from build123d import *

# Parameters (mm, degrees)
BOX319_W                    = 6
BOX319_H                    = 8
BOX319_DEPTH                = 2
BOX319_PLACEMENT_ANGLE      = 45
BOX321_W                    = 6
BOX321_H                    = 8
BOX321_DEPTH                = 2
BOX312_W                    = 6
BOX312_H                    = 8
BOX312_DEPTH                = 2
BOX324_W                    = 6
BOX324_H                    = 8
BOX324_DEPTH                = 2
BOX324_PLACEMENT_ANGLE      = 135
BOX322_W                    = 6
BOX322_H                    = 8
BOX322_DEPTH                = 2
BOX326_W                    = 6
BOX326_H                    = 8
BOX326_DEPTH                = 2
BOX326_PLACEMENT_ANGLE      = 225
BOX315_W                    = 6
BOX315_H                    = 8
BOX315_DEPTH                = 2
BOX325_W                    = 6
BOX325_H                    = 8
BOX325_DEPTH                = 2
BOX325_PLACEMENT_ANGLE      = 45
COMPOUND700_PLACEMENT_ANGLE = 22.5
CYLINDER700_R               = 1.5
CYLINDER700_DEPTH           = 12
CYLINDER700_PLACEMENT_ANGLE = 45
CYLINDER708_R               = 1.5
CYLINDER708_DEPTH           = 12
CYLINDER706_R               = 1.5
CYLINDER706_DEPTH           = 12
CYLINDER706_PLACEMENT_ANGLE = 135
CYLINDER705_R               = 1.5
CYLINDER705_DEPTH           = 12
CYLINDER707_R               = 1.5
CYLINDER707_DEPTH           = 12
CYLINDER707_PLACEMENT_ANGLE = 225
CYLINDER704_R               = 1.5
CYLINDER704_DEPTH           = 12
CYLINDER699_R               = 1.5
CYLINDER699_DEPTH           = 12
CYLINDER699_PLACEMENT_ANGLE = 45
CYLINDER702_R               = 1.5
CYLINDER702_DEPTH           = 12
COMPOUND701_PLACEMENT_ANGLE = 22.5
CYLINDER697_R               = 3.5
CYLINDER697_DEPTH           = 20
TUBE076_R                   = 46
TUBE076_R_2                 = 36
TUBE076_DEPTH               = 1


with BuildPart() as krychle319:
    # Box319 → Box319 (new body)
    with BuildSketch(Plane.XY):
        with Locations((3, 4)):
            Rectangle(BOX319_W, BOX319_H)
    extrude(amount=BOX319_DEPTH)


with BuildPart() as krychle319_1:
    # Box319 placement: moved
    add(krychle319.part.moved(Location((30.405592, -34.648232, 33))).rotate(Axis((30.405592, -34.648232, 33), (0, 0, 1)), BOX319_PLACEMENT_ANGLE))


with BuildPart() as krychle321:
    # Box321 → Box321 (new body)
    with BuildSketch(Plane(origin=(46, -3, 33), x_dir=(0, 1, 0), z_dir=(0, 0, 1))):
        with Locations((3, 4)):
            Rectangle(BOX321_W, BOX321_H)
    extrude(amount=BOX321_DEPTH)


with BuildPart() as krychle312:
    # Box312 → Box312 (new body)
    with BuildSketch(Plane(origin=(-3, -46, 33), x_dir=(1, 0, 0), z_dir=(0, 0, 1))):
        with Locations((3, 4)):
            Rectangle(BOX312_W, BOX312_H)
    extrude(amount=BOX312_DEPTH)


with BuildPart() as krychle324:
    # Box324 → Box324 (new body)
    with BuildSketch(Plane.XY):
        with Locations((3, 4)):
            Rectangle(BOX324_W, BOX324_H)
    extrude(amount=BOX324_DEPTH)


with BuildPart() as krychle324_1:
    # Box324 placement: moved
    add(krychle324.part.moved(Location((34.648232, 30.405592, 33))).rotate(Axis((34.648232, 30.405592, 33), (0, 0, 1)), BOX324_PLACEMENT_ANGLE))


with BuildPart() as krychle322:
    # Box322 → Box322 (new body)
    with BuildSketch(Plane(origin=(3, 46, 33), x_dir=(-1, 0, 0), z_dir=(0, 0, 1))):
        with Locations((3, 4)):
            Rectangle(BOX322_W, BOX322_H)
    extrude(amount=BOX322_DEPTH)


with BuildPart() as krychle326:
    # Box326 → Box326 (new body)
    with BuildSketch(Plane.XY):
        with Locations((3, 4)):
            Rectangle(BOX326_W, BOX326_H)
    extrude(amount=BOX326_DEPTH)


with BuildPart() as krychle326_1:
    # Box326 placement: moved
    add(krychle326.part.moved(Location((-30.405592, 34.648232, 33))).rotate(Axis((-30.405592, 34.648232, 33), (0, 0, 1)), BOX326_PLACEMENT_ANGLE))


with BuildPart() as krychle315:
    # Box315 → Box315 (new body)
    with BuildSketch(Plane(origin=(-46, 3, 33), x_dir=(0, -1, 0), z_dir=(0, 0, 1))):
        with Locations((3, 4)):
            Rectangle(BOX315_W, BOX315_H)
    extrude(amount=BOX315_DEPTH)


with BuildPart() as compound700:
    # Box325 → Box325 (new body)
    with BuildSketch(Plane.XY):
        with Locations((3, 4)):
            Rectangle(BOX325_W, BOX325_H)
    extrude(amount=BOX325_DEPTH)


with BuildPart() as compound700_1:
    # Box325 placement: moved
    add(compound700.part.moved(Location((-34.648232, -30.405592, 33))).rotate(Axis((-34.648232, -30.405592, 33), (0, 0, -1)), BOX325_PLACEMENT_ANGLE))

    # Compound700: union Krychle319, Krychle321, Krychle312, Krychle324, Krychle322, Krychle326, Krychle315
    add(krychle319_1.part)
    add(krychle321.part)
    add(krychle312.part)
    add(krychle324_1.part)
    add(krychle322.part)
    add(krychle326_1.part)
    add(krychle315.part)


with BuildPart() as compound700_2:
    # Compound700 placement: moved
    add(compound700_1.part.rotate(Axis((0, 0, 0), (0, 0, 1)), COMPOUND700_PLACEMENT_ANGLE))


with BuildPart() as obj1:
    # Cylinder700 → Cylinder700 (new body)
    with BuildSketch(Plane.XY):
        Circle(CYLINDER700_R)
    extrude(amount=CYLINDER700_DEPTH)


with BuildPart() as obj1_1:
    # Cylinder700 placement: moved
    add(obj1.part.moved(Location((29.698485, -29.698485, 33.5))).rotate(Axis((29.698485, -29.698485, 33.5), (0, 0, 1)), CYLINDER700_PLACEMENT_ANGLE))


with BuildPart() as obj2:
    # Cylinder708 → Cylinder708 (new body)
    with BuildSketch(Plane(origin=(42, 0, 33.5), x_dir=(0, 1, 0), z_dir=(0, 0, 1))):
        Circle(CYLINDER708_R)
    extrude(amount=CYLINDER708_DEPTH)


with BuildPart() as obj3:
    # Cylinder706 → Cylinder706 (new body)
    with BuildSketch(Plane.XY):
        Circle(CYLINDER706_R)
    extrude(amount=CYLINDER706_DEPTH)


with BuildPart() as obj3_1:
    # Cylinder706 placement: moved
    add(obj3.part.moved(Location((29.698485, 29.698485, 33.5))).rotate(Axis((29.698485, 29.698485, 33.5), (0, 0, 1)), CYLINDER706_PLACEMENT_ANGLE))


with BuildPart() as obj4:
    # Cylinder705 → Cylinder705 (new body)
    with BuildSketch(Plane(origin=(0, 42, 33.5), x_dir=(-1, 0, 0), z_dir=(0, 0, 1))):
        Circle(CYLINDER705_R)
    extrude(amount=CYLINDER705_DEPTH)


with BuildPart() as obj5:
    # Cylinder707 → Cylinder707 (new body)
    with BuildSketch(Plane.XY):
        Circle(CYLINDER707_R)
    extrude(amount=CYLINDER707_DEPTH)


with BuildPart() as obj5_1:
    # Cylinder707 placement: moved
    add(obj5.part.moved(Location((-29.698485, 29.698485, 33.5))).rotate(Axis((-29.698485, 29.698485, 33.5), (0, 0, 1)), CYLINDER707_PLACEMENT_ANGLE))


with BuildPart() as obj6:
    # Cylinder704 → Cylinder704 (new body)
    with BuildSketch(Plane(origin=(-42, 0, 33.5), x_dir=(0, -1, 0), z_dir=(0, 0, 1))):
        Circle(CYLINDER704_R)
    extrude(amount=CYLINDER704_DEPTH)


with BuildPart() as obj7:
    # Cylinder699 → Cylinder699 (new body)
    with BuildSketch(Plane.XY):
        Circle(CYLINDER699_R)
    extrude(amount=CYLINDER699_DEPTH)


with BuildPart() as obj7_1:
    # Cylinder699 placement: moved
    add(obj7.part.moved(Location((-29.698485, -29.698485, 33.5))).rotate(Axis((-29.698485, -29.698485, 33.5), (0, 0, -1)), CYLINDER699_PLACEMENT_ANGLE))


with BuildPart() as compound701:
    # Cylinder702 → Cylinder702 (new body)
    with BuildSketch(Plane(origin=(0, -42, 33.5), x_dir=(1, 0, 0), z_dir=(0, 0, 1))):
        Circle(CYLINDER702_R)
    extrude(amount=CYLINDER702_DEPTH)

    # Compound701: union obj1, obj2, obj3, obj4, obj5, obj6, obj7
    add(obj1_1.part)
    add(obj2.part)
    add(obj3_1.part)
    add(obj4.part)
    add(obj5_1.part)
    add(obj6.part)
    add(obj7_1.part)


with BuildPart() as compound701_1:
    # Compound701 placement: moved
    add(compound701.part.rotate(Axis((0, 0, 0), (0, 0, 1)), COMPOUND701_PLACEMENT_ANGLE))


with BuildPart() as obj8:
    # Cylinder697 → Cylinder697 (new body)
    with BuildSketch(Plane(origin=(-46.3, 0, 29), x_dir=(1, 0, 0), z_dir=(0, 0, 1))):
        Circle(CYLINDER697_R)
    extrude(amount=CYLINDER697_DEPTH)


with BuildPart() as cut321:
    # Tube076 → Tube076 (new body)
    with BuildSketch(Plane.XY.offset(37)):
        Circle(TUBE076_R)
        Circle(TUBE076_R_2, mode=Mode.SUBTRACT)
    extrude(amount=TUBE076_DEPTH)

    # Cut323: cut obj8
    add(obj8.part, mode=Mode.SUBTRACT)

    # Cut330: cut Compound701
    add(compound701_1.part, mode=Mode.SUBTRACT)

    # Cut321: cut Compound700
    add(compound700_2.part, mode=Mode.SUBTRACT)


solid = cut321.part
The listing builds one solid part. Answer for the finished solid, in the listing's coordinates (mm). Give positions to 0.01 mm unless a question says otherwise; leave off trailing zeros. Write each loop counter-clockwise with the first axis right and the second up, starting at its lowest first coordinate (ties: lowest second). Pieces come first, ordered by that corner, then holes.
Item 1: Determine the mould class of faces 1 (the cylindrical face through (-42.8, -0.1, 37.5)), 2 (the flat face through (-27.4, -23.6, 38)), 3 (the cylindrical face through (-16.33, 40.28, 37.49)), 4 (the cylindrical face through (14.844, 37.943, 37.493)) for opening direction X: released by +X, released by -X, zero draft, split by the parting line, or undercut.
Item 2: Flat-ended cylindrical pins translate along their axes: P1, Ø1.8, axis at x = -16.07, y = -38.8, coming from the +Z side; P2, Ø5, axis at x = -38.8, y = 16.07, coming from the +Z side. Find the tip coordinate at first contact, or state that the pin passes through.
Item 3: Section C-C, the plane z = 37.25 is taken. Count the separate pieces of the cut face and the enclosed holes in it, plus the area to 3 significant figures.
Item 4: Find the intervals of material crossed by line 1 along Y through (x, z) = (0.5, 37.5); line 2 along X through (y, z) = (29, 37.45); line 3 along X through (y, z) = (25.5, 37.7), in increasing order.
Item 5: Section B-B, the plane y = 0 is taken. Write down the section's boundary in (x, z).
Item 6: Section A-A, the plane x = 0 is taken. Write down the section's boundary in (y, z).
Completed:
1. face 1: released by -X
1. face 2: zero draft
1. face 3: undercut
1. face 4: undercut
2. P1: passes through
2. P2: stops at z = 38
3. separate pieces: 1
3. enclosed holes: 9
3. area: 2,500 mm2
4. line 1: y = -46 to -36, 36 to 46
4. line 2: x = -35.71 to -21.33, 21.33 to 35.71
4. line 3: x = -38.29 to -25.41, 25.41 to 38.29
5. outline: (-42.8, 37) - (-36, 37) - (-36, 38) - (-42.8, 38) - close; (36, 37) - (46, 37) - (46, 38) - (36, 38) - close
6. outline: (-46, 37) - (-36, 37) - (-36, 38) - (-46, 38) - close; (36, 37) - (46, 37) - (46, 38) - (36, 38) - close
